Geometry check sheet. Reference: the model listing, model coordinates, mm. Round coordinates to 2 decimals unless told otherwise and drop trailing zeros. Return JSON: item names as keys, results as strings. Group by question number.
Q1. Material ranges on line 1 along X through (y, z) = (2, -219); line 2 along X through (y, z) = (9.75, -260); line 3 along Y through (x, z) = (30, -152), recorded low to high.
Q2. Sectioned sample at A-A, the plane z = -172. Give the number of separate pieces and of enclosed holes in the cut face, then the cut area to 3 significant figures.
Q3. Gauge pin test, flat ends, axial feed: pin 1 Ø6 at (y, z) = (13, -25.5) entering from +X; pin 2 Ø4 at (x, z) = (9, -55.5) entering from -Y; pin 3 Ø0.6 at (y, z) = (19, -67.5) entering from +X. Record the tip position at first contact, or that the pin passes through.
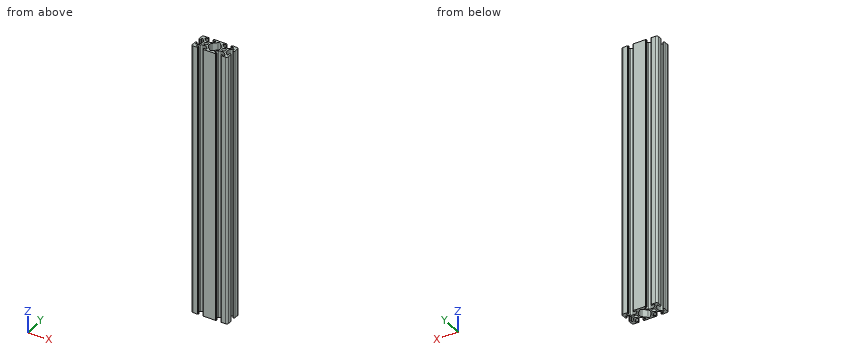
```python
from build123d import *

# Parameters (mm, degrees)
SKIZZE1_R                       = 2.15
AUFSATZ_LINEAR_AUSTRAGEN1_DEPTH = 300


with BuildPart() as part:
    # Skizze1 → Aufsatz-Linear austragen1 (new body)
    with BuildSketch(Plane.XY.offset(20)):
        with BuildLine():
            Line((32.499999987, 1.499999997), (32.499999987, 0.800000002))
            ThreePointArc((32.499999987, 0.800000002), (32.734314563, 0.234314576), (33.29999999, 0))
            Line((33.29999999, 0), (38, 0))
            ThreePointArc((38, 0), (39.414213562, 0.585786438), (40, 2))
            Line((40, 2), (40, 6.700000003))
            ThreePointArc((40, 6.700000003), (39.765685425, 7.265685427), (39.2, 7.500000003))
            Line((39.2, 7.500000003), (38.499999994, 7.500000003))
            ThreePointArc((38.499999994, 7.500000003), (38.28786796, 7.412132037), (38.199999994, 7.200000003))
            Line((38.199999994, 7.200000003), (38.199999994, 5.082411608))
            ThreePointArc((38.199999994, 5.082411608), (37.686138516, 4.313363559), (36.77898449, 4.493807714))
            Line((36.77898449, 4.493807714), (34.52867965, 6.744112554))
            ThreePointArc((34.52867965, 6.744112554), (33.878361397, 7.717382599), (33.649999994, 8.865432896))
            Line((33.649999994, 8.865432896), (33.649999994, 11.134567107))
            ThreePointArc((33.649999994, 11.134567107), (33.878361397, 12.282617403), (34.52867965, 13.255887448))
            Line((34.52867965, 13.255887448), (36.778984494, 15.506192293))
            ThreePointArc((36.778984494, 15.506192293), (37.686138518, 15.686636447), (38.199999994, 14.9175884))
            Line((38.199999994, 14.9175884), (38.199999994, 12.800000003))
            ThreePointArc((38.199999994, 12.800000003), (38.287867961, 12.587867967), (38.499999997, 12.5))
            Line((38.499999997, 12.5), (39.199999998, 12.5))
            ThreePointArc((39.199999998, 12.5), (39.765685424, 12.734314576), (40, 13.300000002))
            Line((40, 13.300000002), (40, 18))
            ThreePointArc((40, 18), (39.414213562, 19.414213562), (38, 20))
            Line((38, 20), (33.299999987, 20))
            ThreePointArc((33.299999987, 20), (32.734314562, 19.765685425), (32.499999987, 19.2))
            Line((32.499999987, 19.2), (32.499999987, 18.499999997))
            ThreePointArc((32.499999987, 18.499999997), (32.587867953, 18.287867963), (32.799999987, 18.199999997))
            Line((32.799999987, 18.199999997), (34.917587987, 18.199999997))
            ThreePointArc((34.917587987, 18.199999997), (35.686635928, 17.686138591), (35.506191799, 16.778984692))
            Line((35.506191799, 16.778984692), (33.255886765, 14.528679659))
            ThreePointArc((33.255886765, 14.528679659), (32.28261672, 13.878361405), (31.134566423, 13.650000003))
            Line((31.134566423, 13.650000003), (28.865432887, 13.650000003))
            ThreePointArc((28.865432887, 13.650000003), (27.717382591, 13.878361405), (26.744112545, 14.528679659))
            Line((26.744112545, 14.528679659), (24.493807705, 16.778984499))
            ThreePointArc((24.493807705, 16.778984499), (24.313363551, 17.686138521), (25.082411597, 18.199999997))
            Line((25.082411597, 18.199999997), (27.199999997, 18.199999997))
            ThreePointArc((27.199999997, 18.199999997), (27.412132033, 18.287867964), (27.5, 18.5))
            Line((27.5, 18.5), (27.5, 19.199999998))
            ThreePointArc((27.5, 19.199999998), (27.265685424, 19.765685424), (26.699999998, 20))
            Line((26.699999998, 20), (13.299999987, 20))
            ThreePointArc((13.299999987, 20), (12.734314562, 19.765685425), (12.499999987, 19.2))
            Line((12.499999987, 19.2), (12.499999987, 18.499999997))
            ThreePointArc((12.499999987, 18.499999997), (12.587867953, 18.287867963), (12.799999987, 18.199999997))
            Line((12.799999987, 18.199999997), (14.917588393, 18.199999997))
            ThreePointArc((14.917588393, 18.199999997), (15.686636443, 17.686138519), (15.506192288, 16.778984492))
            Line((15.506192288, 16.778984492), (13.255887455, 14.528679659))
            ThreePointArc((13.255887455, 14.528679659), (12.282617409, 13.878361405), (11.134567113, 13.650000003))
            Line((11.134567113, 13.650000003), (8.865432887, 13.650000003))
            ThreePointArc((8.865432887, 13.650000003), (7.717382591, 13.878361405), (6.744112545, 14.528679659))
            Line((6.744112545, 14.528679659), (4.493807705, 16.778984499))
            ThreePointArc((4.493807705, 16.778984499), (4.313363551, 17.686138521), (5.082411597, 18.199999997))
            Line((5.082411597, 18.199999997), (7.199999997, 18.199999997))
            ThreePointArc((7.199999997, 18.199999997), (7.412132033, 18.287867964), (7.5, 18.5))
            Line((7.5, 18.5), (7.5, 19.199999998))
            ThreePointArc((7.5, 19.199999998), (7.265685424, 19.765685424), (6.699999997, 20))
            Line((6.699999997, 20), (2, 20))
            ThreePointArc((2, 20), (0.585786438, 19.414213562), (0, 18))
            Line((0, 18), (0, 13.3))
            ThreePointArc((0, 13.3), (0.234314575, 12.734314575), (0.8, 12.5))
            Line((0.8, 12.5), (1.500000005, 12.5))
            ThreePointArc((1.500000005, 12.5), (1.71213204, 12.587867966), (1.800000005, 12.8))
            Line((1.800000005, 12.8), (1.800000005, 14.91758839))
            ThreePointArc((1.800000005, 14.91758839), (2.313861483, 15.686636439), (3.22101551, 15.506192284))
            Line((3.22101551, 15.506192284), (5.471320344, 13.25588745))
            ThreePointArc((5.471320344, 13.25588745), (6.121638597, 12.282617404), (6.35, 11.134567108))
            Line((6.35, 11.134567108), (6.35, 8.86543289))
            ThreePointArc((6.35, 8.86543289), (6.121638597, 7.717382593), (5.471320344, 6.744112548))
            Line((5.471320344, 6.744112548), (3.221015504, 4.493807708))
            ThreePointArc((3.221015504, 4.493807708), (2.313861481, 4.313363554), (1.800000005, 5.0824116))
            Line((1.800000005, 5.0824116), (1.800000005, 7.2))
            ThreePointArc((1.800000005, 7.2), (1.712132039, 7.412132036), (1.500000003, 7.500000003))
            Line((1.500000003, 7.500000003), (0.800000003, 7.500000002))
            ThreePointArc((0.800000003, 7.500000002), (0.234314576, 7.265685427), (0, 6.7))
            Line((0, 6.7), (0, 2))
            ThreePointArc((0, 2), (0.585786438, 0.585786438), (2, 0))
            Line((2, 0), (6.7, 0))
            ThreePointArc((6.7, 0), (7.265685425, 0.234314575), (7.5, 0.8))
            Line((7.5, 0.8), (7.5, 1.5))
            ThreePointArc((7.5, 1.5), (7.412132034, 1.712132034), (7.2, 1.8))
            Line((7.2, 1.8), (5.0824116, 1.8))
            ThreePointArc((5.0824116, 1.8), (4.313363551, 2.313861478), (4.493807706, 3.221015504))
            Line((4.493807706, 3.221015504), (6.744112546, 5.471320344))
            ThreePointArc((6.744112546, 5.471320344), (7.717382592, 6.121638598), (8.865432888, 6.35))
            Line((8.865432888, 6.35), (11.134567107, 6.35))
            ThreePointArc((11.134567107, 6.35), (12.282617403, 6.121638598), (13.255887449, 5.471320344))
            Line((13.255887449, 5.471320344), (15.506192293, 3.2210155))
            ThreePointArc((15.506192293, 3.2210155), (15.686636447, 2.313861477), (14.9175884, 1.8))
            Line((14.9175884, 1.8), (12.79999999, 1.8))
            ThreePointArc((12.79999999, 1.8), (12.587867954, 1.712132033), (12.499999987, 1.499999997))
            Line((12.499999987, 1.499999997), (12.499999987, 0.800000002))
            ThreePointArc((12.499999987, 0.800000002), (12.734314563, 0.234314576), (13.29999999, 0))
            Line((13.29999999, 0), (26.7, 0))
            ThreePointArc((26.7, 0), (27.265685425, 0.234314575), (27.5, 0.8))
            Line((27.5, 0.8), (27.5, 1.5))
            ThreePointArc((27.5, 1.5), (27.412132034, 1.712132034), (27.2, 1.8))
            Line((27.2, 1.8), (25.0824116, 1.8))
            ThreePointArc((25.0824116, 1.8), (24.313363551, 2.313861478), (24.493807706, 3.221015504))
            Line((24.493807706, 3.221015504), (26.744112546, 5.471320344))
            ThreePointArc((26.744112546, 5.471320344), (27.717382592, 6.121638598), (28.865432888, 6.35))
            Line((28.865432888, 6.35), (31.134567114, 6.35))
            ThreePointArc((31.134567114, 6.35), (32.28261741, 6.121638598), (33.255887456, 5.471320344))
            Line((33.255887456, 5.471320344), (35.50619239, 3.22101541))
            ThreePointArc((35.50619239, 3.22101541), (35.686636533, 2.313861444), (34.917588535, 1.8))
            Line((34.917588535, 1.8), (32.79999999, 1.8))
            ThreePointArc((32.79999999, 1.8), (32.587867954, 1.712132033), (32.499999987, 1.499999997))
        make_face()
        with Locations((10, 10)):
            Circle(SKIZZE1_R, mode=Mode.SUBTRACT)
        with Locations((30, 10)):
            Circle(SKIZZE1_R, mode=Mode.SUBTRACT)
        with BuildLine():
            Line((18.585786095, 2.687006109), (14.528679095, 6.744113109))
            ThreePointArc((14.528679095, 6.744113109), (13.878360842, 7.717383154), (13.64999944, 8.86543345))
            Line((13.64999944, 8.86543345), (13.64999944, 11.134566552))
            ThreePointArc((13.64999944, 11.134566552), (13.878360842, 12.282616848), (14.528679095, 13.255886894))
            Line((14.528679095, 13.255886894), (18.585786441, 17.312994239))
            ThreePointArc((18.585786441, 17.312994239), (20.000000001, 17.898780676), (21.414213561, 17.312994239))
            Line((21.414213561, 17.312994239), (25.471320215, 13.255887585))
            ThreePointArc((25.471320215, 13.255887585), (26.121638469, 12.282617539), (26.349999871, 11.134567243))
            Line((26.349999871, 11.134567243), (26.349999871, 8.86543345))
            ThreePointArc((26.349999871, 8.86543345), (26.121638469, 7.717383154), (25.471320215, 6.744113109))
            Line((25.471320215, 6.744113109), (21.414213215, 2.687006109))
            ThreePointArc((21.414213215, 2.687006109), (19.999999655, 2.101219672), (18.585786095, 2.687006109))
        make_face(mode=Mode.SUBTRACT)
    extrude(amount=-AUFSATZ_LINEAR_AUSTRAGEN1_DEPTH)


solid = part.part
```
Reply:
{
 "1": {"line 1": "0 to 4.54, 15.46 to 24.54, 35.46 to 40", "line 2": "6.35 to 7.86, 12.14 to 13.65, 26.35 to 27.86, 32.14 to 33.65", "line 3": "6.35 to 7.85, 12.15 to 13.65"},
 "2": {"separate pieces": "1", "enclosed holes": "3", "area": "332 mm^2"},
 "3": {"pin 1": "x = 40", "pin 2": "y = 0.06", "pin 3": "x = 39.87"}
}
